```python
from build123d import *

# Parameters (mm, degrees)
F0_R     = 18.65
F1_DEPTH = 59
F4_R     = 6
F4_R_2   = 4.6
F5_DEPTH = 22.9
F6_DEPTH = 30.1
F7_DEPTH = 43.9
F8_R     = 20
F8_R_2   = 6
F9_DEPTH = 10


with BuildPart() as f1:
    # F0 (on Front) → F1 (new body)
    with BuildSketch(Plane.XZ):
        Circle(F0_R)
    extrude(amount=-F1_DEPTH)

    # F2 (on Top) → F3 (revolve)
    with BuildSketch(Plane.XY):
        Polygon((23.5, 0), (0, 0), (0, -35), (20.5, -35), (21.6, -3.3), (23.5, -3.3), align=None)
    revolve(axis=Axis((0, -17.5, 0), (0, -1, 0)))

    # F4 (on face) → F5 (join)
    with BuildSketch(Plane.XZ.offset(35)):
        with BuildLine():
            ThreePointArc((12.2, 8.110641), (0, 14.65), (-12.2, 8.110641))
            Line((-12.2, 8.110641), (-12.2, -8.110641))
            ThreePointArc((-12.2, -8.110641), (0, -14.65), (12.2, -8.110641))
            Line((12.2, -8.110641), (12.2, 8.110641))
        make_face()
        Circle(F4_R, mode=Mode.SUBTRACT)
        Circle(F4_R)
        Circle(F4_R_2, mode=Mode.SUBTRACT)
        Circle(F4_R_2)
    extrude(amount=F5_DEPTH)

    # F4 (on face) → F6 (join)
    with BuildSketch(Plane.XZ.offset(35)):
        Circle(F4_R)
        Circle(F4_R_2, mode=Mode.SUBTRACT)
        Circle(F4_R_2)
    extrude(amount=F6_DEPTH)

    # F4 (on face) → F7 (join)
    with BuildSketch(Plane.XZ.offset(35)):
        Circle(F4_R_2)
    extrude(amount=F7_DEPTH)

    # F8 (on face) → F9 (join)
    with BuildSketch(Plane.XZ.offset(65.1)):
        Circle(F8_R)
        Circle(F8_R_2)
    extrude(amount=F9_DEPTH)


solid = f1.part
```
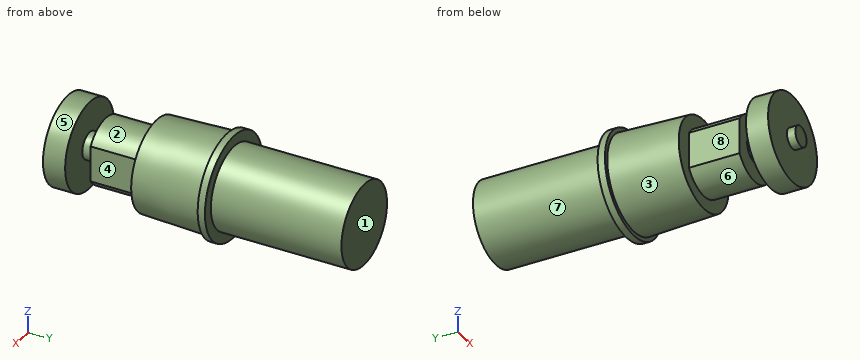
CAD build for the part. Positions are in the model's coordinates, mm. Face numbers are marked on the shaded views. A direction names the side the tool comes from. Round coordinates to 2 decimals unless told otherwise and drop trailing zeros. Order: outer loops, then holes, each group sorted by start corner. A loop starts at its lowest first (then second) coordinate and runs counter-clockwise, first axis right, second up. Notation, with made-up numbers: (82.25, 27.5) - (121.25, 27.5) arc R24 ccw to (121.25, 53.5) - close; hole circle Ø3 at (45, 46). An arc over 180 degrees is marked (long way). Answer in a Markdown table with one row per item. Add a question column.
(1) Drop flat-ended pins along their axis: pin 1 Ø1.5 at (x, z) = (-1.5, 6) entering from -Y; pin 2 Ø12 at (y, z) = (27, 11) entering from +X; pin 3 Ø12 at (x, y) = (-18.5, 10) entering from +Z; pin 4 Ø20.5 at (x, z) = (7, 8.5) entering from -Y. Give the stop position or say it passes through.
(2) Probe L1, parallel to Y at x = 2.5, z = 16; L2, parallel to Y at x = -9.5, z = -6.5; L3, parallel to Y at x = 12.5, z = 18.5. List the from-to ranges inside material, lowest first. Write a range as [from, to].
(3) 3-axis set-ups, long thin cutter, end or side, ignore diameter. For the marked faces 4, 5, 6, 7 and 8: which of +Z, -Z, +X, -X, +Y, -Y reach the whole face in a straight line?
(4) Band-saw the part on D-D on y = 27. List the corners of the cut face in (x, z).
(5) Mould opens along Y. For the marked faces 1, 2 and 3 say: +Y half, -Y half, draft (parallel to the pull), parting line (faces both ways), or undercut.
(6) Band-saw the part on C-C on y = -56.5. List the corners of the cut face in (x, z), and give its area (3 significant figures).
(7) Band-saw the part on A-A on x = 0. List the corners of the cut face in (y, z).
(8) Band-saw the part on B-B on z = 0. List the corners of the cut face in (x, y), and give its area (3 significant figures).
Data:
| question | item | result |
|---|---|---|
| 1 | pin 1 | stops at y = -75.1 |
| 1 | pin 2 | stops at x = 17.97 |
| 1 | pin 3 | stops at z = 13.84 |
| 1 | pin 4 | stops at y = -78.9 |
| 2 | L1 | y = [-75.1, -65.1], [-35, 59] |
| 2 | L2 | y = [-75.1, -65.1], [-57.9, 59] |
| 2 | L3 | y = [-3.3, 0] |
| 3 | face 4 | +Z, -Z, +X |
| 3 | face 5 | -Y |
| 3 | face 6 | -Z |
| 3 | face 7 | +Y |
| 3 | face 8 | +Z, -Z, -X |
| 4 | outline | circle Ø37.3 at (0, 0) |
| 5 | face 1 | +Y half |
| 5 | face 2 | undercut |
| 5 | face 3 | -Y half |
| 6 | outline | (-12.2, -8.11) arc R14.65 ccw to (12.2, -8.11) - (12.2, 8.11) arc R14.65 ccw to (-12.2, 8.11) - close |
| 6 | area | 620 mm^2 |
| 7 | outline | (-78.9, -4.6) - (-75.1, -4.6) - (-75.1, -20) - (-65.1, -20) - (-65.1, -6) - (-57.9, -6) - (-57.9, -14.65) - (-35, -14.65) - (-35, -20.5) - (-3.3, -21.6) - (-3.3, -23.5) - (0, -23.5) - (0, -18.65) - (59, -18.65) - (59, 18.65) - (0, 18.65) - (0, 23.5) - (-3.3, 23.5) - (-3.3, 21.6) - (-35, 20.5) - (-35, 14.65) - (-57.9, 14.65) - (-57.9, 6) - (-65.1, 6) - (-65.1, 20) - (-75.1, 20) - (-75.1, 4.6) - (-78.9, 4.6) - close |
| 8 | outline | (-23.5, -3.3) - (-21.6, -3.3) - (-20.5, -35) - (-12.2, -35) - (-12.2, -57.9) - (-6, -57.9) - (-6, -65.1) - (-20, -65.1) - (-20, -75.1) - (-4.6, -75.1) - (-4.6, -78.9) - (4.6, -78.9) - (4.6, -75.1) - (20, -75.1) - (20, -65.1) - (6, -65.1) - (6, -57.9) - (12.2, -57.9) - (12.2, -35) - (20.5, -35) - (21.6, -3.3) - (23.5, -3.3) - (23.5, 0) - (18.65, 0) - (18.65, 59) - (-18.65, 59) - (-18.65, 0) - (-23.5, 0) - close |
| 8 | area | 4,770 mm^2 |
